Build history of the part. All positions in model axes, mm. A direction names the side the tool comes from. Give positions to 0.01 mm unless a question says otherwise; leave off trailing zeros. Order: outer loops, then holes, each group sorted by start corner. A loop starts at its lowest first (then second) coordinate and runs counter-clockwise, first axis right, second up. Notation, with made-up numbers: (70, 51.5) -> (84, 51.5) arc R17 cw to (84, 80.5) -> close; hole circle Ø6 at (14.25, -21). An arc over 180 degrees is marked (long way). One line per question, with ' | ' between items. Start each with the question number.
(1) Drill centre lines: L1, parallel to Z at x = 0, y = -18; L2, parallel to Z at x = 1.25, y = -10.75; L3, parallel to Y at x = 4.5, z = -6.25. Where is each one in solid material? Low to high. Write a range as from..to.
(2) Which spindle directions (+Z, -Z, +X, -X, +Y, -Y) get a long thin tool onto all of the face, cutting with end or side? Do faces 1 (the face through (3.233, -9.86, -1.341)), 2 (the face through (0, 0, 0)). Say none if no direction does.
(3) Pin check, flat tips, straight feed: pin 1 Ø10 at (y, z) = (-10, -5.5) entering from -X; pin 2 Ø1 at (y, z) = (-21.5, -2.5) entering from +X; pin 3 Ø3 at (x, z) = (4.5, 6) entering from -Y. Stop position of each tip, or through.
(4) Cut at A-A (y = -2). Give the cut face in (x, z), then the cut area to 3 significant figures.
from build123d import *

# Parameters (mm, degrees)
F0_R     = 3.5
F1_DEPTH = 20
F2_R     = 10
F2_R_2   = 3.5
F3_DEPTH = 5


# Not quite as in the source:
# - a fillet or chamfer that OpenCascade refuses, or shapes differently, is made with other operations: its cross-section is extruded or revolved along the edge and cut away or added


with BuildPart() as f1:
    # F0 (on Front) → F1 (new body)
    with BuildSketch(Plane.XZ):
        Circle(F0_R)
    extrude(amount=F1_DEPTH)

    # F2 (on face) → F3 (join)
    with BuildSketch(Plane.XZ.offset(20)):
        Circle(F2_R)
        Circle(F2_R_2, mode=Mode.SUBTRACT)
        Circle(F2_R_2)
    extrude(amount=F3_DEPTH)

    # F4: fillet of radius 10 on 1 edges, made by hand

    # F4_s1 → F4_t2 (revolve, cut)
    with BuildSketch(Plane.XY):
        with BuildLine():
            ThreePointArc((10, -20), (6.3397459622, -23.6602540378), (1.3397459622, -25))
            Line((1.3397459622, -25), (10, -25))
            Line((10, -25), (10, -20))
        make_face()
    revolve(axis=Axis((0, -25, 0), (0, -1, 0)), mode=Mode.SUBTRACT)


solid = f1.part
Result set:
1) L1: z = -3.5..3.5 | L2: z = -3.27..3.27 | L3: y = -22.72..-20
2) face 1: +Y | face 2: +Z, -Z, +X, -X, +Y
3) pin 1: stops at x = -3.46 | pin 2: stops at x = 9.02 | pin 3: stops at y = -23.85
4) outline: circle Ø7 at (0, 0) | area: 38.5 mm2
